```python
from build123d import *

# Parameters (mm, degrees)
F1_DEPTH = 2000


with BuildPart() as f1:
    # F0 (on Front) → F1 (new body)
    with BuildSketch(Plane.XZ):
        with BuildLine():
            Line((-17.24309, -5.361117), (-15.74309, -5.361117))
            Line((-15.74309, -5.361117), (-15.74309, 10.638883))
            ThreePointArc((-15.74309, 10.638883), (-16.914663, 13.46731), (-19.74309, 14.638883))
            Line((-19.74309, 14.638883), (-38.24309, 14.638883))
            ThreePointArc((-38.24309, 14.638883), (-40.010857, 15.371116), (-40.74309, 17.138883))
            Line((-40.74309, 17.138883), (-40.74309, 1009.138883))
            ThreePointArc((-40.74309, 1009.138883), (-40.010857, 1010.90665), (-38.24309, 1011.638883))
            Line((-38.24309, 1011.638883), (-22.24309, 1011.638883))
            Line((-22.24309, 1011.638883), (-22.24309, 1013.138883))
            Line((-22.24309, 1013.138883), (-38.24309, 1013.138883))
            ThreePointArc((-38.24309, 1013.138883), (-41.071517, 1011.96731), (-42.24309, 1009.138883))
            Line((-42.24309, 1009.138883), (-42.24309, 17.138883))
            ThreePointArc((-42.24309, 17.138883), (-41.071517, 14.310456), (-38.24309, 13.138883))
            Line((-38.24309, 13.138883), (-19.74309, 13.138883))
            ThreePointArc((-19.74309, 13.138883), (-17.975323, 12.40665), (-17.24309, 10.638883))
            Line((-17.24309, 10.638883), (-17.24309, -5.361117))
        make_face()
    extrude(amount=F1_DEPTH)


solid = f1.part
```
Input: part model. Units: mm. Frame: model coordinates. Coordinates: 2 decimals unless noted, no trailing zeros. Loops run counter-clockwise (first coordinate to the right, second up) from the corner with the lowest first, then second, coordinate; pieces in that order, holes last. Notation, with made-up numbers: (-40, -37.5) -> (10, -37.5) arc R9 ccw to (10, -30.5) -> close; hole circle Ø3 at (70, 66). An arc over 180 degrees is marked (long way). Use a Markdown table: item, result.
1) Pull-direction query (Z, two-part tool) for faces 1 (the flat face through (-42.243, -986, 520)), 2 (the flat face through (-40.743, -986, 506)); classes: released by +Z, released by -Z, zero draft, split by the parting line, or undercut.
Results found:
| item | result |
|---|---|
| face 1 | zero draft |
| face 2 | undercut |
2) Cut plane B-B (y = -854.5). Return the cut outline in (x, z), then the cut area to 3 significant figures.
Results found:
| item | result |
|---|---|
| outline | (-42.24, 17.14) arc R4 ccw to (-38.24, 13.14) -> (-19.74, 13.14) arc R2.5 cw to (-17.24, 10.64) -> (-17.24, -5.36) -> (-15.74, -5.36) -> (-15.74, 10.64) arc R4 ccw to (-19.74, 14.64) -> (-38.24, 14.64) arc R2.5 cw to (-40.74, 17.14) -> (-40.74, 1009.14) arc R2.5 cw to (-38.24, 1011.64) -> (-22.24, 1011.64) -> (-22.24, 1013.14) -> (-38.24, 1013.14) arc R4 ccw to (-42.24, 1009.14) -> close |
| area | 1,590 mm2 |
3) Cut plane C-C (z = 241). Return the cut outline in (x, y), then the cut area to 3 significant figures.
Results found:
| item | result |
|---|---|
| outline | (-42.24, -2000) -> (-40.74, -2000) -> (-40.74, 0) -> (-42.24, 0) -> close |
| area | 3,000 mm2 |
4) Cut plane A-A (x = -28.75). Return the cut outline in (y, z).
Results found:
| item | result |
|---|---|
| outline | (-2000, 13.14) -> (0, 13.14) -> (0, 14.64) -> (-2000, 14.64) -> close; (-2000, 1011.64) -> (0, 1011.64) -> (0, 1013.14) -> (-2000, 1013.14) -> close |
5) Material intervals for line 1 along Z through (x, y) = (-29, -1246.5); line 2 along X through (y, z) = (-1174, 137.5); line 3 along Z through (x, y) = (-40.25, -1732.5), sorted ascending. Write a range as from..to.
Results found:
| item | result |
|---|---|
| line 1 | z = 13.14..14.64, 1011.64..1013.14 |
| line 2 | x = -42.24..-40.74 |
| line 3 | z = 13.68..15.65, 1010.63..1012.6 |
6) Contact query for flat-ended pins moving along their axis: pin 1 (15 mm diameter, centred on x = -31, y = -1188, fed in from -Z); pin 2 (17.5 mm diameter, centred on y = -1242, z = 2.5, fed in from -X); pin 3 (3 mm diameter, centred on y = -794, z = 203.5, fed in from +X). Output: stop coordinate, or through.
Results found:
| item | result |
|---|---|
| pin 1 | stops at z = 13.14 |
| pin 2 | stops at x = -17.32 |
| pin 3 | stops at x = -40.74 |
